Part model, mm, in its own coordinate system. Face numbers are marked on the shaded views. A direction names the side the tool comes from. Give positions to 0.01 mm unless a question says otherwise; leave off trailing zeros. Write each loop counter-clockwise with the first axis right and the second up, starting at its lowest first coordinate (ties: lowest second). Pieces come first, ordered by that corner, then holes. Notation, with made-up numbers: M 34,37.5 L 79,37.5 A20 cw 79,58.5 Z; hole C 28,2.5 d4. An arc over 180 degrees is marked long. Use CSV: the item, a comma, the result in double quotes. Start each with the question number.
1. Mould opens along X. For the marked faces 1, 2, 3 and 4 say: pulls with the +X half, pulls with the -X half, needs draft (parallel to the pull), parting line crosses it, or undercut.
2. Band-saw the part on B-B, the plane y = -38.5. List the corners of the cut face in (x, z).
3. 3-axis set-ups, long thin cutter, end or side, ignore diameter. For the marked faces 5 and 6: which of +Z, -Z, +X, -X, +Y, -Y reach the whole face in a straight line?
4. Band-saw the part on A-A, the plane y = -21.59. List the corners of the cut face in (x, z).
5. Drop flat-ended pins along their axis: pin 1 Ø4.5 at (x, y) = (136, -21.5) entering from +Z; pin 2 Ø10 at (y, z) = (-37, 28) entering from -X; pin 3 Ø4 at (y, z) = (-35, 15.5) entering from +X. Give the stop position or say it passes through.
6. Drill centre lines: line 1 along Z through (x, y) = (141, -6); line 2 along X through (y, z) = (-23, 23); line 3 along X through (y, z) = (-30.5, 29). Where is each one in solid material? Low to high. Write a range as from..to.
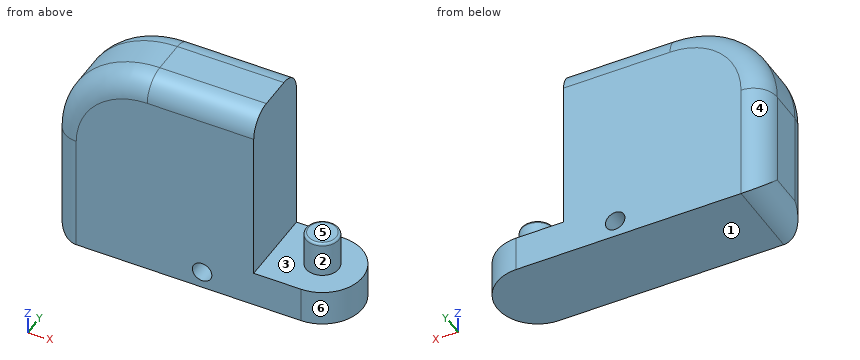
from build123d import *

# Parameters (mm, degrees)
F0_W     = 25.4
F0_H     = 19.304
F1_DEPTH = 43.18
F3_DEPTH = 19.304
F4_R     = 8.763
F5_DEPTH = 19.304
F6_R     = 1.27
F7_R     = 12.7
F8_R     = 5.2197
F9_DEPTH = 43.181


with BuildPart() as f1:
    # F0 (on Front) → F1 (new body)
    with BuildSketch(Plane.XZ):
        with BuildLine():
            Line((0, 63.5), (0, 0))
            Line((0, 0), (107.95, 0))
            Line((107.95, 0), (107.95, 19.304))
            Line((107.95, 19.304), (107.95, 114.3))
            Line((107.95, 114.3), (50.8, 114.3))
            ThreePointArc((50.8, 114.3), (14.878976, 99.421024), (0, 63.5))
        make_face()
        with Locations((120.65, 9.652)):
            Rectangle(F0_W, F0_H)
    extrude(amount=F1_DEPTH)

    # F2 (on face) → F3 (join)
    with BuildSketch(Plane.XY.offset(19.304)):
        with BuildLine():
            Line((133.35, 0), (133.35, -43.18))
            ThreePointArc((133.35, -43.18), (154.94, -21.59), (133.35, 0))
        make_face()
    extrude(amount=-F3_DEPTH)

    # F4 (on face) → F5 (join)
    with BuildSketch(Plane.XY.offset(19.304)):
        with Locations((133.35, -21.59)):
            Circle(F4_R)
    extrude(amount=F5_DEPTH)

    # F6
    f6_edges = [f1.edges().sort_by_distance(p)[0] for p in [
        (124.587, -21.59, 38.608),
    ]]
    fillet(f6_edges, radius=F6_R)

    # F7
    f7_edges = [f1.edges().sort_by_distance(p)[0] for p in [
        (50.8, -21.59, 114.3),
        (0, -21.59, 63.5),
        (14.878976, 0, 99.421024),
        (14.878976, -43.18, 99.421024),
        (0, -21.59, 0),
    ]]
    fillet(f7_edges, radius=F7_R)

    # F8 (on face) → F9 (cut, through all)
    with BuildSketch(Plane.XZ.offset(43.18)):
        with Locations((80.242619, 9.295693)):
            Circle(F8_R)
    extrude(amount=-F9_DEPTH, mode=Mode.SUBTRACT)


solid = f1.part
Output:
1,face 1,"needs draft"
1,face 2,"undercut"
1,face 3,"undercut"
1,face 4,"pulls with the -X half"
2,outline,"M 2.85,4.68 A12.7 ccw 12.7,0 L 146.77,0 L 146.77,19.3 L 107.95,19.3 L 107.95,111.45 L 50.8,111.45 A47.95 ccw 2.85,63.5 Z; hole C 80.24,9.3 d10.44"
3,face 5,"+Z, +X, +Y, -Y"
3,face 6,"+Z, -Z, +X"
4,outline,"M 0,12.7 A12.7 ccw 12.7,0 L 154.94,0 L 154.94,19.3 L 142.11,19.3 L 142.11,37.34 A1.27 ccw 140.84,38.61 L 125.86,38.61 A1.27 ccw 124.59,37.34 L 124.59,19.3 L 107.95,19.3 L 107.95,114.3 L 50.8,114.3 A50.8 ccw 0,63.5 Z; hole C 80.24,9.3 d10.44"
5,pin 1,"stops at z = 38.61"
5,pin 2,"stops at x = 0.09"
5,pin 3,"stops at x = 151.68"
6,line 1,"z = 0..19.3"
6,line 2,"x = 0..107.95, 124.7..142"
6,line 3,"x = 0..107.95"
